Autodesk Inventor part; units mm, degrees
ref_plane "YZ Plane" through (0, 0, 0) normal (1, 0, 0) x (0, 1, 0)
ref_plane "XZ Plane" through (0, 0, 0) normal (0, 1, 0) x (-1, 0, 0)
ref_plane "XY Plane" through (0, 0, 0) normal (0, 0, 1) x (1, 0, 0)
sketch "Sketch1" plane through (0, 0, 0) normal (0, 0, 1) x (1, 0, 0)
  line L0 (3.175, 0) -> (3.175, 3.175)
  line L1 (3.175, 3.175) -> (-3.175, 3.175)
  line L2 (-3.175, 3.175) -> (-3.175, 0)
  line L3 (-5.08, 0) -> (-5.08, 5.08)
  line L4 (-5.08, 5.08) -> (5.08, 5.08)
  line L5 (5.08, 5.08) -> (5.08, 0)
  line L6 (5.08, 0) -> (3.175, 0)
  line L7 (-3.175, 0) -> (-5.08, 0)
  point P0 (0, 0)
  dimension "d0" = 10.16
  dimension "d1" = 5.08
extrude "Extrusion1" add sketch "Sketch1" along normal blind 368.3
sketch "Sketch2" plane through (-5.08, 5.08, 0) normal (0, 1, 0) x (1, 0, 0)
  circle A0 centre (5.08, -6.35) radius 1.9844
  circle A1 centre (5.08, -44.45) radius 1.9844
  circle A2 centre (5.08, -361.95) radius 1.9844
  circle A3 centre (5.08, -323.85) radius 1.9844
  point P0 (5.08, 0)
  dimension "d4" = 3.9688
  dimension "d5" = 3.9688
  dimension "d6" = 3.9688
  dimension "d7" = 3.9688
extrude "Extrusion2" cut sketch "Sketch2" against normal blind 368.3
sketch "Sketch3" plane through (0, 0, 0) normal (0, 0, -1) x (-1, 0, 0)
  line L0 (-5.08, 0) -> (-5.08, 5.08)
  line L1 (5.08, 5.08) -> (-5.08, 5.08)
  line L2 (-5.08, 5.08) -> (-5.08, 0)
  line L3 (-5.08, 0) -> (5.08, 0)
  line L4 (5.08, 0) -> (5.08, 5.08)
  point P0 (0, 0)
sketch "Sketch4" plane through (0, 0, 0) normal (0, 0, -1) x (-1, 0, 0)
  point P0 (0, 0)
extrude "Extrusion3" add sketch "Sketch3" along normal blind 1.778
sketch "Sketch5" plane through (-5.08, 5.08, 368.3) normal (0, 1, 0) x (1, 0, 0)
  circle A0 centre (5.08, 6.35) radius 1.9844
  circle A1 centre (5.08, 44.45) radius 1.9844
  circle A2 centre (5.08, 323.85) radius 1.9844
  circle A3 centre (5.08, 361.95) radius 1.9844
  circle A4 centre (5.08, 6.35) radius 5.08
  line L0 (10.16, 0) -> (10.16, 370.078)
  circle A5 centre (5.08, 44.45) radius 5.08
  circle A6 centre (5.08, 323.85) radius 5.08
  circle A7 centre (5.08, 361.95) radius 5.08
  point P0 (5.08, 368.3)
extrude "Extrusion4" add sketch "Sketch5" along normal blind 6.35
sketch "Sketch6" plane through (0, 0, 368.3) normal (0, 0, 1) x (1, 0, 0)
  line L0 (-15.875, -1.5875) -> (12.7, -1.5875)
  line L1 (12.7, -1.5875) -> (12.7, 14.2875)
  line L2 (12.7, 14.2875) -> (-15.875, 14.2875)
  line L3 (-15.875, 14.2875) -> (-15.875, -1.5875)
  point P0 (0, 0)
extrude "Extrusion5" cut sketch "Sketch6" against normal blind 184.15
properties part number "hs_intake_cb_jig_second"
Check sheet for the modelled part. Datum: model origin and axes. Units: mm. A direction names the side the tool comes from. Coordinates: 2 decimals unless noted, no trailing zeros. Write each loop counter-clockwise with the first axis right and the second up, starting at its lowest first coordinate (ties: lowest second). Pieces come first, ordered by that corner, then holes. Notation, with made-up numbers: (66.25, 52) - (123.25, 52) arc R17 cw to (123.25, 57) - close; hole circle Ø4 at (-13, 72.5). An arc over 180 degrees is marked (long way). One line per question, with ' | ' between items.
Item 1: Access from +Z, -Z, +X, -X, +Y, -Y to the whole of each face (thin tool, end or side, straight path). Record for faces 4 (the face through (-1.1, 8.21, 1.39)), 5 (the face through (0, 5.08, 1)), 6 (the face through (5.08, 3, 92)), 7 (the face through (0, 2, 0)).
Determined:
face 4: +Y | face 5: -Z, +Y | face 6: +Z, -Z, +X, +Y, -Y | face 7: +Z, -Y
Item 2: Thickness scan on line 1 (Z direction, x = 0, y = 7.25); line 2 (X direction, y = 2.5, z = 52) (3 decimals); line 3 (X direction, y = 7.5, z = 6.35). Record the ranges inside material, lowest first. Write a range as [from, to].
Determined:
line 1: z = [1.27, 4.37], [8.33, 11.43], [39.37, 42.47], [46.43, 49.53] | line 2: x = [-5.08, -3.175], [3.175, 5.08] | line 3: x = [-5.08, -1.98], [1.98, 5.08]
Item 3: Sectioned sample at B-B on z = 70.5. Record the boundary of the cut face in (x, y) (3 decimals).
Determined:
outline: (-5.08, 0) - (-3.175, 0) - (-3.175, 3.175) - (3.175, 3.175) - (3.175, 0) - (5.08, 0) - (5.08, 5.08) - (-5.08, 5.08) - close
Item 4: Sectioned sample at A-A on x = 0. Record the boundary of the cut face in (y, z) (3 decimals), plus the area to 3 significant figures.
Determined:
outline: (0, -1.778) - (5.08, -1.778) - (5.08, 1.27) - (11.43, 1.27) - (11.43, 4.366) - (3.175, 4.366) - (3.175, 0) - (0, 0) - close; (3.175, 8.334) - (11.43, 8.334) - (11.43, 11.43) - (5.08, 11.43) - (5.08, 39.37) - (11.43, 39.37) - (11.43, 42.466) - (3.175, 42.466) - close; (3.175, 46.434) - (11.43, 46.434) - (11.43, 49.53) - (5.08, 49.53) - (5.08, 184.15) - (3.175, 184.15) - close | area: 423 mm2
Item 5: Gauge pin test, flat ends, axial feed: P1, Ø1.6, axis at x = -0.5, y = 2, coming from the +Z side; P2, Ø3, axis at x = 0, z = 67.5, coming from the -Y side (3 decimals); P3, Ø2, axis at x = 3, y = 8, coming from the -Z side. Record the tip position at first contact, or that the pin passes through.
Determined:
P1: stops at z = 0 | P2: stops at y = 3.175 | P3: stops at z = 1.68
Item 6: Mould release check, pull along Z, two halves, no side actions. Record for faces 1 (the face through (0, 5.08, 26)), 2 (the face through (0, 3.175, 91)), 3 (the face through (0, 4, 184.15)): pulls with the +Z half, pulls with the -Z half, needs draft (parallel to the pull), parting line crosses it, or undercut.
Determined:
face 1: undercut | face 2: needs draft | face 3: pulls with the +Z half
